from build123d import *

# Parameters (mm, degrees)
CYLINDER1671_R              = 1.5
CYLINDER1671_DEPTH          = 20
CYLINDER1670_R              = 1.5
CYLINDER1670_DEPTH          = 20
COMPOUND820_ROLL_ANGLE      = 90
COMPOUND820_PLACEMENT_ANGLE = 90
CYLINDER1622_R              = 1.5
CYLINDER1622_DEPTH          = 60
CYLINDER1623_R              = 1.5
CYLINDER1623_DEPTH          = 60
CYLINDER1624_R              = 1.5
CYLINDER1624_DEPTH          = 60
CYLINDER1621_R              = 1.5
CYLINDER1621_DEPTH          = 60
CYLINDER1629_R              = 4
CYLINDER1629_DEPTH          = 48
BOX656_W                    = 42
BOX656_H                    = 32
BOX656_DEPTH                = 1
CHAMFER046_SIZE             = 4


with BuildPart() as obj1:
    # Cylinder1671 → Cylinder1671 (new body)
    with BuildSketch(Plane(origin=(15.75, 114, 58.525), x_dir=(-1, 0, 0), z_dir=(0, 1, 0))):
        Circle(CYLINDER1671_R)
    extrude(amount=CYLINDER1671_DEPTH)


with BuildPart() as compound821:
    # Cylinder1670 → Cylinder1670 (new body)
    with BuildSketch(Plane(origin=(15.75, 114, 39.48), x_dir=(-1, 0, 0), z_dir=(0, 1, 0))):
        Circle(CYLINDER1670_R)
    extrude(amount=CYLINDER1670_DEPTH)

    # Compound820: union obj1
    add(obj1.part)


with BuildPart() as compound821_1:
    # Compound820 roll: moved
    add(compound821.part.rotate(Axis((0, 0, 0), (1, 0, 0)), COMPOUND820_ROLL_ANGLE))


with BuildPart() as compound821_2:
    # Compound820 placement: moved
    add(compound821_1.part.moved(Location((-49, 0, -96))).rotate(Axis((-49, 0, -96), (0, 0, 1)), COMPOUND820_PLACEMENT_ANGLE))


with BuildPart() as compound821_3:
    # Compound821 placement: moved
    add(compound821_2.part.moved(Location((0, 74, -80))))


with BuildPart() as obj2:
    # Cylinder1622 → Cylinder1622 (new body)
    with BuildSketch(Plane(origin=(18, 85, -57), x_dir=(1, 0, 0), z_dir=(0, 0, 1))):
        Circle(CYLINDER1622_R)
    extrude(amount=CYLINDER1622_DEPTH)


with BuildPart() as obj3:
    # Cylinder1623 → Cylinder1623 (new body)
    with BuildSketch(Plane(origin=(-18, 85, -57), x_dir=(1, 0, 0), z_dir=(0, 0, 1))):
        Circle(CYLINDER1623_R)
    extrude(amount=CYLINDER1623_DEPTH)


with BuildPart() as obj4:
    # Cylinder1624 → Cylinder1624 (new body)
    with BuildSketch(Plane(origin=(-18, 95, -57), x_dir=(1, 0, 0), z_dir=(0, 0, 1))):
        Circle(CYLINDER1624_R)
    extrude(amount=CYLINDER1624_DEPTH)


with BuildPart() as compound806:
    # Cylinder1621 → Cylinder1621 (new body)
    with BuildSketch(Plane(origin=(18, 95, -57), x_dir=(1, 0, 0), z_dir=(0, 0, 1))):
        Circle(CYLINDER1621_R)
    extrude(amount=CYLINDER1621_DEPTH)

    # Compound806: union obj2, obj3, obj4
    add(obj2.part)
    add(obj3.part)
    add(obj4.part)


with BuildPart() as obj5:
    # Cylinder1629 → Cylinder1629 (new body)
    with BuildSketch(Plane(origin=(0, 90, -55), x_dir=(1, 0, 0), z_dir=(0, 0, 1))):
        Circle(CYLINDER1629_R)
    extrude(amount=CYLINDER1629_DEPTH)


with BuildPart() as chamfer046:
    # Box656 → Box656 (new body)
    with BuildSketch(Plane(origin=(-21, 80, -49), x_dir=(1, 0, 0), z_dir=(0, 0, 1))):
        with Locations((21, 16)):
            Rectangle(BOX656_W, BOX656_H)
    extrude(amount=BOX656_DEPTH)

    # Cut318: cut obj5
    add(obj5.part, mode=Mode.SUBTRACT)

    # Cut320: cut Compound806
    add(compound806.part, mode=Mode.SUBTRACT)

    # Cut333: cut Compound821
    add(compound821_3.part, mode=Mode.SUBTRACT)

    # Chamfer046
    chamfer046_edges = [chamfer046.edges().sort_by_distance(p)[0] for p in [
        (-21, 112, -48.5),
        (21, 112, -48.5),
    ]]
    chamfer(chamfer046_edges, length=CHAMFER046_SIZE)


solid = chamfer046.part
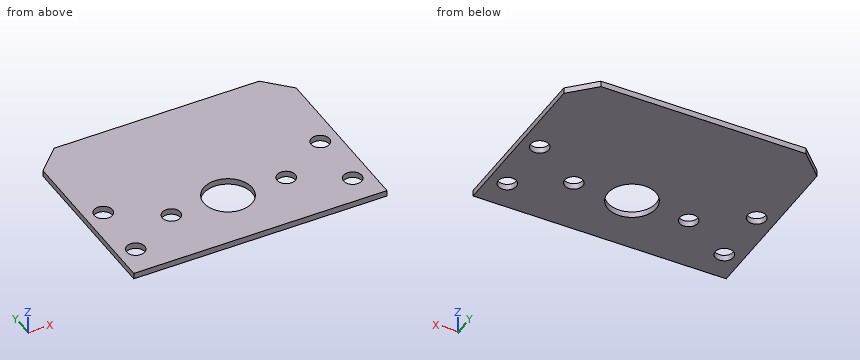
The listing builds one solid part. Answer for the finished solid, in the listing's coordinates (mm). Coordinates: 2 decimals unless noted, no trailing zeros. Loops run counter-clockwise (first coordinate to the right, second up) from the corner with the lowest first, then second, coordinate; pieces in that order, holes last. Notation, with made-up numbers: (-36, 87) -> (-3, 87) arc R19 cw to (-3, 95) -> close; hole circle Ø3 at (-9, 63.25). An arc over 180 degrees is marked (long way). Answer in a Markdown table with one row per item. Add a question column.
1. The part is cut by section D-D, the plane z = -48.65. Write down the section's boundary in (x, y) (3 decimals), then the cut area to 3 significant figures.
2. The part is cut by section B-B, the plane y = 85. Write down the section's boundary in (x, z).
3. The part is cut by section C-C, the plane y = 90. Write down the section's boundary in (x, z).
4. The part is cut by section A-A, the plane x = -9.52. Write down the section's boundary in (y, z), then the cut area to 3 significant figures.
5. Consider line 1 (X direction, y = 85, z = -48.5); line 2 (X direction, y = 89.75, z = -48.6) (3 decimals); line 3 (Y direction, x = 18, z = -48.35). Determine where each line is inside the solid, lowest interval first. Write a range as [from, to].
Answer below:
| question | item | result |
|---|---|---|
| 1 | outline | (-21, 80) -> (21, 80) -> (21, 108) -> (17, 112) -> (-17, 112) -> (-21, 108) -> close; hole circle Ø3 at (-18, 85); hole circle Ø3 at (-18, 95); hole circle Ø3 at (-9.52, 89.75); hole circle Ø8 at (0, 90); hole circle Ø3 at (9.525, 89.75); hole circle Ø3 at (18, 85); hole circle Ø3 at (18, 95) |
| 1 | area | 1,240 mm2 |
| 2 | outline | (-21, -49) -> (-19.5, -49) -> (-19.5, -48) -> (-21, -48) -> close; (-16.5, -49) -> (16.5, -49) -> (16.5, -48) -> (-16.5, -48) -> close; (19.5, -49) -> (21, -49) -> (21, -48) -> (19.5, -48) -> close |
| 3 | outline | (-21, -49) -> (-11, -49) -> (-11, -48) -> (-21, -48) -> close; (-8.04, -49) -> (-4, -49) -> (-4, -48) -> (-8.04, -48) -> close; (4, -49) -> (8.05, -49) -> (8.05, -48) -> (4, -48) -> close; (11, -49) -> (21, -49) -> (21, -48) -> (11, -48) -> close |
| 4 | outline | (80, -49) -> (88.25, -49) -> (88.25, -48) -> (80, -48) -> close; (91.25, -49) -> (112, -49) -> (112, -48) -> (91.25, -48) -> close |
| 4 | area | 29.0 mm2 |
| 5 | line 1 | [-21, -19.5], [-16.5, 16.5], [19.5, 21] |
| 5 | line 2 | [-21, -11.02], [-8.02, -3.992], [3.992, 8.025], [11.025, 21] |
| 5 | line 3 | [80, 83.5], [86.5, 93.5], [96.5, 111] |
